Could you check a few things on this model? Use its own coordinates, in mm. Face numbers are marked on the shaded views. Round coordinates to 2 decimals unless told otherwise and drop trailing zeros. Loops run counter-clockwise (first coordinate to the right, second up) from the corner with the lowest first, then second, coordinate; pieces in that order, holes last.
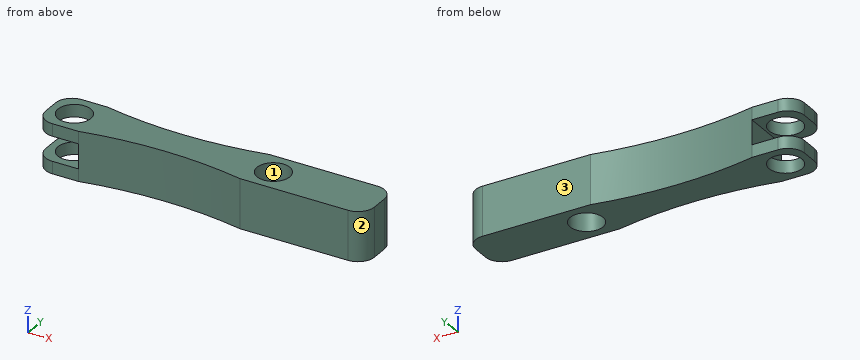
from build123d import *

# Parameters (mm, degrees)
SKETCH1_W           = 200
SKETCH1_H           = 30
BOSS_EXTRUDE1_DEPTH = 30
FILLET1_R           = 10
CUT_EXTRUDE1_DEPTH  = 30
SKETCH4_W           = 15
SKETCH4_H           = 30
CUT_EXTRUDE3_DEPTH  = 26
SKETCH5_R           = 10
CUT_EXTRUDE4_DEPTH  = 45
SCALE1_SCALE        = 4


with BuildPart() as part:
    # Sketch1 → Boss-Extrude1 (new body)
    with BuildSketch(Plane.XY):
        with Locations((46.259717806, -4.797058824)):
            Rectangle(SKETCH1_W, SKETCH1_H)
    extrude(amount=BOSS_EXTRUDE1_DEPTH)

    # Fillet1
    fillet1_edges = [part.edges().sort_by_distance(p)[0] for p in [
        (-53.740282194, 10.202941176, 15),
        (146.259717806, 10.202941176, 15),
        (146.259717806, -19.797058824, 15),
        (-53.740282194, -19.797058824, 15),
    ]]
    fillet(fillet1_edges, radius=FILLET1_R)

    # Sketch2 → Cut-Extrude1 (cut)
    with BuildSketch(Plane.XY.offset(30)):
        with BuildLine():
            Line((-27.901084514, 10.202941176), (70.420520136, 10.202941176))
            ThreePointArc((70.420520136, 10.202941176), (21.259717811, 5.202941178), (-27.901084514, 10.202941176))
        make_face()
        with BuildLine():
            Line((-27.901084524, -19.797058824), (70.420520136, -19.797058824))
            ThreePointArc((70.420520136, -19.797058824), (21.259717806, -14.798405243), (-27.901084524, -19.797058824))
        make_face()
    extrude(amount=-CUT_EXTRUDE1_DEPTH, mode=Mode.SUBTRACT)

    # Sketch4 → Cut-Extrude3 (cut)
    with BuildSketch(Plane.ZY.offset(53.740282194)):
        with Locations((15, -4.797058824)):
            Rectangle(SKETCH4_W, SKETCH4_H)
    extrude(amount=-CUT_EXTRUDE3_DEPTH, mode=Mode.SUBTRACT)

    # Sketch5 → Cut-Extrude4 (cut)
    with BuildSketch(Plane.XY.offset(30)):
        with Locations((-39.286224807, -4.797058824)):
            Circle(SKETCH5_R)
        with Locations((81.809717806, -4.797058824)):
            Circle(SKETCH5_R)
    extrude(amount=-CUT_EXTRUDE4_DEPTH, mode=Mode.SUBTRACT)


with BuildPart() as part_1:
    # Scale1: scaled about (57.695562261, -4.797279973, 15)
    add(part.part.scale(SCALE1_SCALE).moved(Location((-173.086686783, 14.391839919, -45))))


solid = part_1.part
Item 1: If I drill on line 1 along X through (y, z) = (-1.5, 14.5); line 2 along X through (y, z) = (25, -28); line 3 along X through (y, z) = (17, -18.5), over which ranges is the centre line in solid material (lowest first)?
Results list:
line 1: x = -284.05 to 114.29, 194.02 to 411.95
line 2: x = -386.83 to -356.92, -303.54 to 127.47, 180.84 to 410.73
line 3: x = -388.01 to -363.77, -296.69 to 120.61, 187.69 to 411.91
Item 2: If we section it at B-B, the plane x = 146: Please give me the cut outline in (y, z), then the cut area to 3 significant figures.
Results list:
outline: (-64.8, -45) - (-43.96, -45) - (-43.96, 75) - (-64.8, 75) - close; (34.36, -45) - (55.2, -45) - (55.2, 75) - (34.36, 75) - close
area: 5,000 mm2
Item 3: If we section it at A-A, the plane z = 64.5: Please give me the cut outline in (x, y), then the cut area to 3 significant figures.
Results list:
outline: (-388.05, -24.8) arc R40 ccw to (-348.05, -64.8) - (-284.69, -64.8) arc R976.97 cw to (108.6, -64.8) - (371.95, -64.8) arc R40 ccw to (411.95, -24.8) - (411.95, 15.2) arc R40 ccw to (371.95, 55.2) - (108.6, 55.2) arc R976.71 cw to (-284.69, 55.2) - (-348.05, 55.2) arc R40 ccw to (-388.05, 15.2) - close; hole circle Ø80 at (-330.23, -4.8); hole circle Ø80 at (154.15, -4.8)
area: 74,100 mm2
Item 4: If we section it at D-D, the plane x = -335: Please give me the cut outline in (y, z).
Results list:
outline: (-64.8, -45) - (-44.51, -45) - (-44.51, -15) - (-64.8, -15) - close; (-64.8, 45) - (-44.51, 45) - (-44.51, 75) - (-64.8, 75) - close; (34.92, -45) - (55.2, -45) - (55.2, -15) - (34.92, -15) - close; (34.92, 45) - (55.2, 45) - (55.2, 75) - (34.92, 75) - close
Item 5: Will these pins go through, and if not, where does the flat tip stop? pin 1 (2 mm diameter, centred on y = 20, z = -20.5, fed in from -X); pin 2 (10 mm diameter, centred on x = -21.5, z = 21, fed in from +Y); pin 3 (2 mm diameter, centred on x = -37, y = -48.5, fed in from -Z); pin 4 (8 mm diameter, centred on y = 30, z = -27.5, fed in from +X).
Results list:
pin 1: stops at x = -387.87
pin 2: stops at y = 37.83
pin 3: passes through
pin 4: stops at x = 410.47
Item 6: We'd pull the mould along X, two halves only. Please class the marked faces 1, 2 and 3: released by +X, released by -X, zero draft, split by the parting line, or undercut.
Results list:
face 1: undercut
face 2: released by +X
face 3: zero draft
Item 7: If we section it at C-C, the plane z = 19: Please give me the cut outline in (x, y), then the cut area to 3 significant figures.
Results list:
outline: (-284.05, -64.66) arc R976.97 cw to (108.6, -64.8) - (371.95, -64.8) arc R40 ccw to (411.95, -24.8) - (411.95, 15.2) arc R40 ccw to (371.95, 55.2) - (108.6, 55.2) arc R976.71 cw to (-284.05, 55.07) - close; hole circle Ø80 at (154.15, -4.8)
area: 67,300 mm2
